Input: part model. Units: mm. Frame: model coordinates. A direction names the side the tool comes from. Give positions to 0.01 mm unless a question says otherwise; leave off trailing zeros. Loops run counter-clockwise (first coordinate to the right, second up) from the corner with the lowest first, then second, coordinate; pieces in that order, holes last. Notation, with made-up numbers: (52.25, -12.5) -> (80.25, -12.5) arc R21 cw to (80.25, 10.5) -> close; hole circle Ø6 at (-20, -5.5). An arc over 180 degrees is marked (long way). One line per question, with ' | ' between items.
Autodesk Inventor part; units mm, degrees
ref_plane "YZ Plane" through (0, 0, 0) normal (1, 0, 0) x (0, 1, 0)
ref_plane "XZ Plane" through (0, 0, 0) normal (0, 1, 0) x (-1, 0, 0)
ref_plane "XY Plane" through (0, 0, 0) normal (0, 0, 1) x (1, 0, 0)
sketch "Sketch1" plane through (0, 0, 0) normal (0, 0, 1) x (1, 0, 0)
  line L0 (3.6662, 6.35) -> (7.3323, 0)
  line L1 (7.3323, 0) -> (3.6662, -6.35)
  line L2 (3.6662, -6.35) -> (-3.6662, -6.35)
  line L3 (-3.6662, -6.35) -> (-7.3323, 0)
  line L4 (-7.3323, 0) -> (-3.6662, 6.35)
  line L5 (-3.6662, 6.35) -> (3.6662, 6.35)
  circle A0 centre (0, 0) radius 2.0193
  dimension "d0" = 12.7
  dimension "d3" = 4.0386
extrude "Extrusion2" add sketch "Sketch1" along normal mid plane 63.5
sketch "Sketch2" plane through (0, 0, 31.75) normal (0, 0, 1) x (1, 0, 0)
  point P0 (0, 0)
  point P1 (0, 0)
hole "Hole1" at (0, 0, 31.75) direction (0, 0, -1) diameter 5.842 depth 7.874 counterbore diameter 6.096 counterbore depth 6.1239
sketch "Sketch3" plane through (0, 0, -31.75) normal (0, 0, -1) x (-1, 0, 0)
  point P0 (0, 0)
  point P1 (0, 0)
hole "Hole2" at (0, 0, -31.75) direction (0, 0, 1) diameter 5.842 depth 7.874 counterbore diameter 6.096 counterbore depth 6.1239
properties part number "1_2 x 2_500-inchHexShaft"
1. Section query C-C (y = 4). Output: boundary loops of the cut face in (x, z).
Determined:
outline: (-5.02, -31.75) -> (5.02, -31.75) -> (5.02, 31.75) -> (-5.02, 31.75) -> close
2. Reachability of faces 1 (the flat face through (-5.474, -3.219, -0.444)), 2 (the cylindrical face through (-3.02, -0.4, -28.65)), 3 (the cylindrical face through (2.852, 0.633, 24.739)) from +Z, -Z, +X, -X, +Y, -Y: full face, straight path, thin tool, end or side. Return the list, or none.
Determined:
face 1: +Z, -Z, -X, -Y | face 2: -Z | face 3: +Z
3. Pin query (flat end, axial travel): P1, Ø3, axis at y = -1, z = -18.5, coming from the +X side; P2, Ø3, axis at x = 0, y = 0, coming from the -Z side; P3, Ø4, axis at y = 3, z = -5, coming from the +X side; P4, Ø1, axis at x = 5, z = 12.5, coming from the +Y side. Return the tip coordinate at first contact, or that it passes through.
Determined:
P1: stops at x = 7.33 | P2: passes through | P3: stops at x = 6.75 | P4: stops at y = 4.91
4. Section query B-B (z = 10.5). Output: boundary loops of the cut face in (x, y), then the cut area to 3 significant figures.
Determined:
outline: (-7.33, 0) -> (-3.67, -6.35) -> (3.67, -6.35) -> (7.33, 0) -> (3.67, 6.35) -> (-3.67, 6.35) -> close; hole circle Ø4.04 at (0, 0) | area: 127 mm2
5. Ray query, line 1 along X through (y, z) = (0, 24.75); line 2 along Y through (x, z) = (0, -24.7); line 3 along X through (y, z) = (0, 9). Return the intervals inside material, ascending. Write a range as from..to.
Determined:
line 1: x = -7.33..-2.92, 2.92..7.33 | line 2: y = -6.35..-2.92, 2.92..6.35 | line 3: x = -7.33..-2.02, 2.02..7.33
6. Section query A-A (x = 0). Output: boundary loops of the cut face in (y, z), then the cut area to 3 significant figures.
Determined:
outline: (-6.35, -31.75) -> (-3.05, -31.75) -> (-3.05, -25.63) -> (-2.92, -25.63) -> (-2.92, -23.88) -> (-2.02, -23.88) -> (-2.02, 23.88) -> (-2.92, 23.88) -> (-2.92, 25.63) -> (-3.05, 25.63) -> (-3.05, 31.75) -> (-6.35, 31.75) -> close; (2.02, -23.88) -> (2.92, -23.88) -> (2.92, -25.63) -> (3.05, -25.63) -> (3.05, -31.75) -> (6.35, -31.75) -> (6.35, 31.75) -> (3.05, 31.75) -> (3.05, 25.63) -> (2.92, 25.63) -> (2.92, 23.88) -> (2.02, 23.88) -> close | area: 518 mm2
7. Pull-direction query (X, two-part tool) for faces 4 (the flat face through (0, 6.35, 0)), 5 (the cylindrical face through (1.926, -0.607, -0.334)), 6 (the flat face through (5.525, -3.131, -0.444)); classes: pulls with the +X half, pulls with the -X half, needs draft (parallel to the pull), parting line crosses it, or undercut.
Determined:
face 4: needs draft | face 5: undercut | face 6: pulls with the +X half
